Could you check a few things on this model? Use its own coordinates, in mm. A direction names the side the tool comes from. Coordinates: 2 decimals unless noted, no trailing zeros. Write each loop counter-clockwise with the first axis right and the second up, starting at its lowest first coordinate (ties: lowest second). Pieces come first, ordered by that corner, then holes.
```python
from build123d import *

# Parameters (mm, degrees)
SKETCH1_W           = 406.4
SKETCH1_H           = 406.4
BOSS_EXTRUDE1_DEPTH = 12.7
CUT_EXTRUDE1_DEPTH  = 6.35
SKETCH3_R           = 14.2875
CUT_EXTRUDE2_DEPTH  = 13.7
SKETCH4_R           = 3.175
CUT_EXTRUDE3_DEPTH  = 13.7


with BuildPart() as part:
    # Sketch1 → Boss-Extrude1 (new body)
    with BuildSketch(Plane.XY):
        Rectangle(SKETCH1_W, SKETCH1_H)
    extrude(amount=BOSS_EXTRUDE1_DEPTH)

    # Sketch2 → Cut-Extrude1 (cut)
    with BuildSketch(Plane(origin=(0, 0, 0), x_dir=(-1, 0, 0), z_dir=(0, 0, -1))):
        with BuildLine():
            Line((17.696900373, 168.938120694), (18.027683557, 172.095842576))
            ThreePointArc((18.027683557, 172.095842576), (-128.571850923, -115.806975422), (173.0375, 0))
            Line((173.0375, 0), (173.0375, 203.2))
            Line((173.0375, 203.2), (169.8625, 203.2))
            Line((169.8625, 203.2), (169.8625, 0))
            ThreePointArc((169.8625, 0), (-126.212734393, -113.68207679), (17.696900373, 168.938120694))
        make_face()
    extrude(amount=-CUT_EXTRUDE1_DEPTH, mode=Mode.SUBTRACT)

    # Sketch3 → Cut-Extrude2 (cut, through all)
    with BuildSketch(Plane(origin=(0, 0, 0), x_dir=(-1, 0, 0), z_dir=(0, 0, -1))):
        with BuildLine():
            ThreePointArc((203.2, 0), (143.684097941, -143.684097933), (1.1e-08, -203.2))
            Line((1.1e-08, -203.2), (203.2, -203.2))
            Line((203.2, -203.2), (203.2, 0))
        make_face()
        with BuildLine():
            ThreePointArc((1.1e-08, -203.2), (-143.684098268, -143.684097606), (-203.2, 9.47e-07))
            Line((-203.2, 9.47e-07), (-203.2, -203.2))
            Line((-203.2, -203.2), (1.1e-08, -203.2))
        make_face()
        with BuildLine():
            ThreePointArc((-203.2, 9.47e-07), (-163.039512773, 121.278016454), (-58.432704894, 194.617211466))
            Line((-58.432704894, 194.617211466), (-58.432704894, 203.2))
            Line((-58.432704894, 203.2), (-203.2, 203.2))
            Line((-203.2, 203.2), (-203.2, 9.47e-07))
        make_face()
        Circle(SKETCH3_R)
    extrude(amount=-CUT_EXTRUDE2_DEPTH, mode=Mode.SUBTRACT)

    # Sketch4 → Cut-Extrude3 (cut, through all)
    with BuildSketch(Plane(origin=(0, 0, 0), x_dir=(-1, 0, 0), z_dir=(0, 0, -1))):
        with Locations((-164.977839421, -95.25)):
            Circle(SKETCH4_R)
        with Locations((0, 190.5)):
            Circle(SKETCH4_R)
        with Locations((164.977839421, -95.25)):
            Circle(SKETCH4_R)
        with Locations((190.5, 190.5)):
            Circle(SKETCH4_R)
    extrude(amount=-CUT_EXTRUDE3_DEPTH, mode=Mode.SUBTRACT)


solid = part.part
```
Item 1: If we mould it in two halves opening along Y, with no side actions, what happens to faces 1 (the flat face through (-203.2, 100, 6)), 2 (the flat face through (-74, 203.2, 6)), 3 (the cylindrical face through (122.31, -117.87, 3.13))? For each: released by +Y, released by -Y, zero draft, split by the parting line, or undercut.
Item 2: If I drill on line 1 along Y through (x, z) = (0, 4) (1 decimal); line 2 along Y through (x, z) = (0, 6.75) (1 decimal); line 3 along X through (y, z) = (-112, 1.75), over which ranges is the centre line in solid material (lowest first)?
Item 3: Will these pins go through, and if not, where does the flat tip stop? pin 1 Ø5 at (x, y) = (0, 190.5) entering from +Z; pin 2 Ø1 at (x, z) = (126, 10.5) entering from +Y; pin 3 Ø2 at (y, z) = (110, 7) entering from +X; pin 4 Ø5 at (y, z) = (-129.5, 8.5) entering from +X.
Item 4: Which directions (+Z, -Z, +X, -X, +Y, -Y) give clear straight access to the entire face, cutting with the end or side of a thin tool? Please do faces 4 (the cylindrical face through (132.4, -111.41, 3.13)), 5 (the flat face through (-3, 48, 12.7)).
Item 5: I want a section at C-C, the plane x = 42. List the corners of the cut face in (y, z) for me, then the cut area to 3 significant figures.
Item 6: I want a section at B-B, the plane y = 116. List the corners of the cut face in (x, z) for me, then the cut area to 3 significant figures.
Item 7: I want a section at A-A, the plane z = 4. Count the separate pieces of the cut face and the enclosed holes in it, then the cut area to 3 significant figures.
Taken from the geometry:
1. face 1: zero draft
1. face 2: released by +Y
1. face 3: undercut
2. line 1: y = -203.2 to -173, -169.9 to -14.3, 14.3 to 169.9, 173 to 187.3, 193.7 to 203.2
2. line 2: y = -203.2 to -14.3, 14.3 to 187.3, 193.7 to 203.2
2. line 3: x = -169.55 to -131.9, -127.71 to 127.71, 131.9 to 169.55
3. pin 1: passes through
3. pin 2: stops at y = 159.81
3. pin 3: stops at x = 171.49
3. pin 4: stops at x = 158.62
4. face 4: -Z
4. face 5: +Z, +X, -X, +Y, -Y
5. outline: (-198.81, 0) - (-167.86, 0) - (-167.86, 6.35) - (-164.59, 6.35) - (-164.59, 0) - (164.59, 0) - (164.59, 6.35) - (167.86, 6.35) - (167.86, 0) - (203.2, 0) - (203.2, 12.7) - (-198.81, 12.7) - close
5. area: 5,060 mm2
6. outline: (-203.2, 0) - (-173.04, 0) - (-173.04, 6.35) - (-169.86, 6.35) - (-169.86, 0) - (124.09, 0) - (124.09, 6.35) - (128.4, 6.35) - (128.4, 0) - (166.84, 0) - (166.84, 12.7) - (-203.2, 12.7) - close
6. area: 4,650 mm2
7. separate pieces: 1
7. enclosed holes: 5
7. area: 135,000 mm2
